Autodesk Inventor part; units mm, degrees
ref_plane "YZ Plane" through (0, 0, 0) normal (1, 0, 0) x (0, 1, 0)
ref_plane "XZ Plane" through (0, 0, 0) normal (0, 1, 0) x (-1, 0, 0)
ref_plane "XY Plane" through (0, 0, 0) normal (0, 0, 1) x (1, 0, 0)
sketch "Sketch1" plane through (0, 0, 0) normal (0, 1, 0) x (-1, 0, 0)
  line L0 (3.175, 0) -> (47.625, 0)
  line L1 (50.8, -3.175) -> (50.8, -123.825)
  line L2 (47.625, -127) -> (3.175, -127)
  line L3 (0, -123.825) -> (0, -3.175)
  arc A0 (50.8, -3.175) -> (47.625, 0) centre (47.625, -3.175) ccw
  arc A1 (3.175, 0) -> (0, -3.175) centre (3.175, -3.175) ccw
  arc A2 (0, -123.825) -> (3.175, -127) centre (3.175, -123.825) ccw
  arc A3 (47.625, -127) -> (50.8, -123.825) centre (47.625, -123.825) ccw
  point P0 (0, 0)
  point P1 (50.8, -127)
  point P2 (50.8, 0)
  point P3 (0, -127)
  dimension "d0" = 50.8
  dimension "d1" = 127
  dimension "d4" = 3.175
extrude "Extrusion1" add sketch "Sketch1" along normal blind 12.7
sketch "Sketch2" plane through (0, 12.7, 0) normal (0, 1, 0) x (1, 0, 0)
  line L0 (0, 0) -> (-6.35, 0) construction
  line L1 (-6.35, 0) -> (-6.35, 6.35) construction
  line L2 (-6.35, 6.35) -> (0, 6.35) construction
  line L3 (0, 6.35) -> (0, 0) construction
  circle A0 centre (-6.35, 6.35) radius 3.175
  line L4 (0, 3.175) -> (0, 123.825) construction
  line L5 (0, 63.5) -> (-50.8802, 63.5) construction
  line L6 (-50.8802, 63.5) -> (-25.4, 127) construction
  line L7 (-3.175, 127) -> (-47.625, 127) construction
  line L8 (-25.4, 127) -> (-25.4, 0) construction
  line L9 (-47.625, 0) -> (-3.175, 0) construction
  circle A1 centre (-6.35, 120.65) radius 3.175
  circle A2 centre (-44.45, 6.35) radius 3.175
  circle A3 centre (-44.45, 120.65) radius 3.175
  dimension "d5" = 6.35
  dimension "d6" = 6.35
  dimension "d7" = 6.35
extrude "Extrusion2" cut sketch "Sketch2" against normal through all
sketch "Sketch3" plane through (0, 12.7, 0) normal (0, 1, 0) x (1, 0, 0)
  line L0 (0, 0) -> (-12.7, 0) construction
  line L1 (0, 0) -> (12.7, 0) construction
  line L2 (-47.625, 0) -> (-3.175, 0) construction
  line L3 (-25.4, 0) -> (-25.4, 127) construction
  line L4 (-3.175, 127) -> (-47.625, 127) construction
  line L5 (-50.8, 0) -> (-38.1, 0) construction
  line L6 (-38.1, 0) -> (-12.7, 0)
  line L7 (-12.7, 0) -> (-12.7, 127)
  line L8 (-12.7, 127) -> (-38.1, 127)
  line L9 (-38.1, 127) -> (-38.1, 0)
  dimension "d14" = 12.7
  dimension "d15" = 180
  dimension "d36" = 25.4
extrude "Extrusion3" add sketch "Sketch3" along normal blind 63.5
sketch "Sketch5" plane through (-12.7, 12.7, 0) normal (1, 0, 0) x (0, 0, -1)
  line L0 (0, 63.5) -> (127, 63.5) construction
  line L1 (63.5, 63.5) -> (63.5, 0) construction
  line L2 (123.825, 0) -> (3.175, 0) construction
  line L3 (127, 0) -> (127, 63.5) construction
  circle A0 centre (63.5, 31.7498) radius 6.35
  circle A1 centre (12.7, 31.7498) radius 6.35
  circle A2 centre (114.3, 31.7498) radius 6.35
  line L4 (0, 0) -> (0, 63.5) construction
  line L5 (0, 31.75) -> (127, 31.75) construction
  point P0 (0, -12.7)
  dimension "d24" = 12.7
  dimension "d27" = 12.7
  dimension "d37" = 50.8
  dimension "d38" = 50.8
extrude "Extrusion5" cut sketch "Sketch5" against normal blind 12.7
sketch "Sketch6" plane through (0, 12.7, 0) normal (0, 1, 0) x (1, 0, 0)
  line L0 (-12.7, 0) -> (-19.05, 0)
  line L1 (-19.05, 0) -> (-19.05, 19.05)
  line L2 (-19.05, 19.05) -> (-12.7, 19.05)
  line L3 (-12.7, 19.05) -> (-12.7, 0)
  line L4 (-38.1, 127) -> (-38.1, 0) construction
  line L5 (-38.4604, 63.7403) -> (-13.0604, 63.7086) construction
  line L6 (-12.7, 69.85) -> (-12.7, 57.15) construction
  line L7 (-12.541, 127.416) -> (-18.891, 127.4319)
  line L8 (-18.891, 127.4319) -> (-18.9385, 108.3819)
  line L9 (-18.9385, 108.3819) -> (-12.5885, 108.3661)
  line L10 (-12.5885, 108.3661) -> (-12.541, 127.416)
  line L11 (-47.625, 0) -> (-3.175, 0) construction
  line L12 (-25.4, 0) -> (-25.4, 127) construction
  line L13 (-3.175, 127) -> (-47.625, 127) construction
  line L14 (-38.1, 0) -> (-31.75, 0)
  line L15 (-31.75, 0) -> (-31.75, 19.05)
  line L16 (-31.75, 19.05) -> (-38.1, 19.05)
  line L17 (-38.1, 19.05) -> (-38.1, 0)
  line L18 (-38.1, 69.85) -> (-38.1, 57.15) construction
  line L19 (-38.259, 127.416) -> (-31.909, 127.4319)
  line L20 (-31.909, 127.4319) -> (-31.8615, 108.3819)
  line L21 (-31.8615, 108.3819) -> (-38.2115, 108.3661)
  line L22 (-38.2115, 108.3661) -> (-38.259, 127.416)
  line L23 (-47.625, 0) -> (-2.456, 0) construction
  point P0 (0, 0)
  point P1 (-37.7396, 63.7086)
  point P2 (-38.1, 69.85)
  point P3 (-38.1, 57.15)
  dimension "d30" = 6.35
  dimension "d31" = 19.05
extrude "Extrusion6" cut sketch "Sketch6" along normal blind 8.382
sketch "Sketch7" plane through (0, 0, 0) normal (0, -1, 0) x (1, 0, 0)
  line L0 (-3.175, 0) -> (-47.625, 0) construction
  line L1 (-50.8, -3.175) -> (-50.8, -123.825) construction
  line L2 (-47.625, -127) -> (-3.175, -127) construction
  line L3 (0, -123.825) -> (0, -3.175) construction
  circle A0 centre (-44.45, -6.35) radius 3.175 construction
  circle A1 centre (-44.45, -6.35) radius 3.175 construction
  circle A2 centre (-6.35, -6.35) radius 3.175 construction
  circle A3 centre (-6.35, -6.35) radius 3.175 construction
  circle A4 centre (-44.45, -120.65) radius 3.175 construction
  circle A5 centre (-44.45, -120.65) radius 3.175 construction
  circle A6 centre (-6.35, -120.65) radius 3.175 construction
  arc A7 (-47.625, 0) -> (-50.8, -3.175) centre (-47.625, -3.175) ccw construction
  arc A8 (0, -3.175) -> (-3.175, 0) centre (-3.175, -3.175) ccw construction
  arc A9 (-3.175, -127) -> (0, -123.825) centre (-3.175, -123.825) ccw construction
  arc A10 (-50.8, -123.825) -> (-47.625, -127) centre (-47.625, -123.825) ccw construction
  point P0 (0, 0)
  dimension "d39" = 3.175
properties part number "Far Gantry Bracket"
Here's how the part is built. I have some questions about the finished solid (model axes, mm). A direction names the side the tool comes from. Coordinates: 2 decimals unless noted, no trailing zeros. Order: outer loops, then holes, each group sorted by start corner. A loop starts at its lowest first (then second) coordinate and runs counter-clockwise, first axis right, second up. Notation, with made-up numbers: (17.5, 44.25) - (56.5, 44.25) arc R29 cw to (56.5, 74.25) - close; hole circle Ø1 at (15, -29). An arc over 180 degrees is marked (long way). One line per question, with ' | ' between items. Start each with the question number.
1. If we section it at A-A (x = -6.35): Write out the boundary of the cut face in (y, z) (3 decimals).
2. If we mould it in two halves opening along Z, with no side actions, what happens to faces 1 (the cylindrical face through (-0.95, 6.26, -126.09)), 2 (the cylindrical face through (-7.04, 6.44, -117.55)), 3 (the flat face through (-35, 17, -19.05)), 4 (the flat face through (-38.1, 44, -64))? For each: released by +Z, released by -Z, zero draft, split by the parting line, or undercut.
3. If we section it at C-C (z = -34): Write out the boundary of the cut face in (x, y).
4. I'm going to push flat-ended pins straight in: pin 1 Ø7.5 at (y, z) = (44.45, -63.5) entering from +X; pin 2 Ø6.5 at (y, z) = (18, -6) entering from +X; pin 3 Ø7.5 at (x, z) = (-44.45, -6.35) entering from +Y. Where does each tip first touch, or does it pass through?
5. Which directions (+Z, -Z, +X, -X, +Y, -Y) give clear straight access to the entire face, cutting with the end or side of a thin tool? Please do faces 5 (the cylindrical face through (-18.96, 48.74, -8.02)), 6 (the flat face through (-35, 21.082, -118)), 7 (the flat face through (-16, 21.082, -118)).
6. If we section it at B-B (y = 11): Write out the boundary of the cut face in (x, z) (3 decimals), and give its area (3 significant figures).
7. If we section it at D-D (x = -22): Write out the boundary of the cut face in (y, z).
8. Please list where these lines run through material, in increasing order: line 1 along Z through (x, y) = (-6.35, 5.5) (3 decimals); line 2 along Y through (x, z) = (-16, -114); line 3 along X through (y, z) = (9, -6). Write a range as [from, to].
Model answer:
1) outline: (0, -127) - (12.7, -127) - (12.7, -123.825) - (0, -123.825) - close; (0, -117.475) - (12.7, -117.475) - (12.7, -9.525) - (0, -9.525) - close; (0, -3.175) - (12.7, -3.175) - (12.7, 0) - (0, 0) - close
2) face 1: released by -Z | face 2: undercut | face 3: released by +Z | face 4: zero draft
3) outline: (-50.8, 0) - (0, 0) - (0, 12.7) - (-12.7, 12.7) - (-12.7, 76.2) - (-38.1, 76.2) - (-38.1, 12.7) - (-50.8, 12.7) - close
4) pin 1: stops at x = -25.4 | pin 2: stops at x = -12.7 | pin 3: stops at y = 12.7
5) face 5: +X | face 6: -Z, -X | face 7: -Z, +X
6) outline: (-50.8, -123.825) arc R3.175 ccw to (-47.625, -127) - (-3.175, -127) arc R3.175 ccw to (0, -123.825) - (0, -3.175) arc R3.175 ccw to (-3.175, 0) - (-47.625, 0) arc R3.175 ccw to (-50.8, -3.175) - close; hole circle Ø6.35 at (-44.45, -120.65); hole circle Ø6.35 at (-44.45, -6.35); hole circle Ø6.35 at (-6.35, -120.65); hole circle Ø6.35 at (-6.35, -6.35) | area: 6,320 mm²
7) outline: (0, -127) - (76.2, -127) - (76.2, 0) - (0, 0) - close; hole circle Ø12.7 at (44.45, -114.3); hole circle Ø12.7 at (44.45, -63.5); hole circle Ø12.7 at (44.45, -12.7)
8) line 1: z = [-127, -123.825], [-117.475, -9.525], [-3.175, 0] | line 2: y = [0, 12.7], [21.08, 38.11], [50.79, 76.2] | line 3: x = [-50.8, -47.61], [-41.29, -9.51], [-3.19, 0]
